Geometry: final body of the model. Coordinates: model frame, mm. A direction names the side the tool comes from. Coordinates: 2 decimals unless noted, no trailing zeros. Order: outer loops, then holes, each group sorted by start corner. A loop starts at its lowest first (then second) coordinate and runs counter-clockwise, first axis right, second up. Notation, with made-up numbers: (39.5, 38.25) -> (79.5, 38.25) arc R21 ccw to (79.5, 76.25) -> close; hole circle Ø3 at (88.5, 72.5). An arc over 180 degrees is marked (long way). Answer in a Markdown table with one row per item. Add a question column.
1) Ray query, line 1 (Y direction, x = 132.5, z = 5.25); line 2 (Z direction, x = 136.75, y = 84); line 3 (Y direction, x = 86, z = 5.25). Return the intervals inside material, ascending. Write a range as from..to.
2) Section query C-C on x = 60.5. Return the cut outline in (y, z), then the cut area to 3 significant figures.
3) Contact query for flat-ended pins moving along their axis: P1, Ø1, axis at x = 112, z = 3, coming from the +Y side; P2, Ø6, axis at y = 84, z = 5, coming from the -X side; P3, Ø3, axis at y = 83.5, z = 6, coming from the +X side. Output: stop coordinate, or through.
4) Section query B-B on y = 74.5. Return the cut outline in (x, z).
5) Pull-direction query (Z, two-part tool) for faces 4 (the face through (89, 34, 10)), 5 (the face through (44.9, 86.5, 5.1)), 6 (the face through (89, 70, 5)), 7 (the face through (134.9, 86.5, 5.1)); classes: +Z half, -Z half, draft (parallel to the pull), parting line (faces both ways), or undercut.
6) Set-up query: faces 1 (the face through (160, 70, 5)), 2 (the face through (20, 70, 5)), 3 (the face through (135, 88, 9)). Return all of +Z, -Z, +X, -X, +Y, -Y with unobstructed straight access to the full face (end or side cutting, diameter ignored); none if empty.
```python
from build123d import *

# Parameters (mm, degrees)
F0_W     = 180
F0_H     = 70
F1_DEPTH = 10
F3_W     = 10
F3_H     = 10
F4_DEPTH = 20
F5_R     = 2.5
F6_DEPTH = 140.001
F7_R     = 4.99999
F8_SIZE  = 3


# Not quite as in the source:
# - a fillet or chamfer is up to 0.001 mm smaller than in the source, because OpenCascade refuses the exact size


with BuildPart() as f1:
    # F0 (on Top) → F1 (new body)
    with BuildSketch(Plane.XY):
        with Locations((90, 35)):
            Rectangle(F0_W, F0_H)
    extrude(amount=F1_DEPTH)

    # F3 (on face) → F4 (join)
    with BuildSketch(Plane(origin=(0, 70, 0), x_dir=(-1, 0, 0), z_dir=(0, 1, 0))):
        with Locations((-135, 5)):
            Rectangle(F3_W, F3_H)
        with Locations((-45, 5)):
            Rectangle(F3_W, F3_H)
    extrude(amount=F4_DEPTH)

    # F5 (on face) → F6 (cut, through all)
    with BuildSketch(Plane(origin=(40, 0, 0), x_dir=(0, -1, 0), z_dir=(-1, 0, 0))):
        with Locations((-84, 5)):
            Circle(F5_R)
    extrude(amount=-F6_DEPTH, mode=Mode.SUBTRACT)

    # F7 (radius 5 in the source; OpenCascade refuses exactly that, so slightly less here)
    f7_edges = [f1.edges().sort_by_distance(p)[0] for p in [
        (135, 90, 10),
        (135, 90, 0),
        (45, 90, 0),
        (45, 90, 10),
    ]]
    fillet(f7_edges, radius=F7_R)

    # F8
    f8_edges = [f1.edges().sort_by_distance(p)[0] for p in [
        (90, 70, 10),
        (20, 70, 10),
        (160, 70, 10),
        (160, 70, 0),
        (90, 70, 0),
        (20, 70, 0),
    ]]
    chamfer(f8_edges, length=F8_SIZE)


solid = f1.part
```
Result:
| question | item | result |
|---|---|---|
| 1 | line 1 | 0..81.51, 86.49..89.99 |
| 1 | line 2 | 0..2.5, 7.5..10 |
| 1 | line 3 | 0..70 |
| 2 | outline | (0, 0) -> (67, 0) -> (70, 3) -> (70, 7) -> (67, 10) -> (0, 10) -> close |
| 2 | area | 691 mm2 |
| 3 | P1 | y = 70 |
| 3 | P2 | x = 40 |
| 3 | P3 | x = 140 |
| 4 | outline | (40, 0) -> (50, 0) -> (50, 10) -> (40, 10) -> close; (130, 0) -> (140, 0) -> (140, 10) -> (130, 10) -> close |
| 5 | face 4 | +Z half |
| 5 | face 5 | undercut |
| 5 | face 6 | draft |
| 5 | face 7 | undercut |
| 6 | face 1 | +Z, -Z, +X, +Y |
| 6 | face 2 | +Z, -Z, -X, +Y |
| 6 | face 3 | +Z, +X, -X, +Y |
